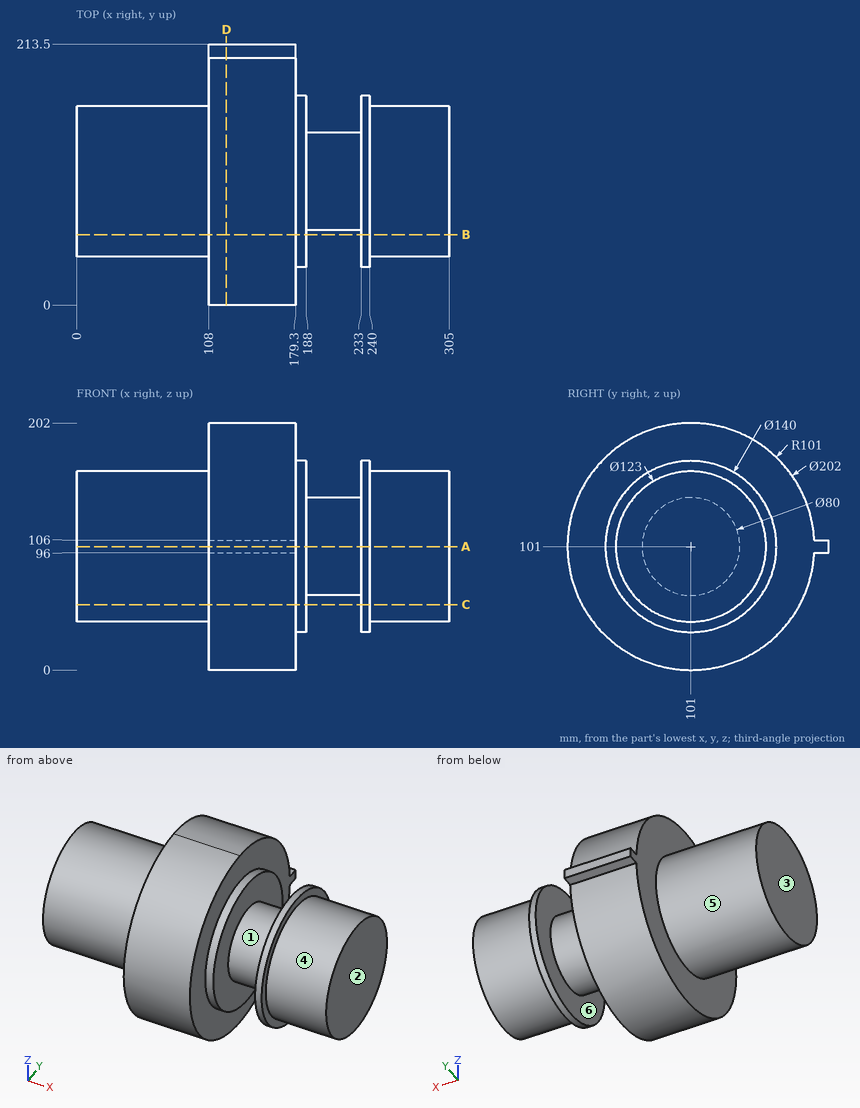
Study the drawing (mm; zero at the part's minimum x, y, z) and answer. A direction names the side the tool comes from. Give positions to 0.01 mm unless a question says otherwise; leave off trailing zeros. Write each loop counter-clockwise with the first axis right and the second up, starting at its lowest first coordinate (ties: lowest second). Pieces come first, ordered by that corner, then holes. Notation, with made-up numbers: (41.25, 76) - (47.25, 76) arc R34 ccw to (47.25, 111) - close; hole circle Ø4 at (33, 23). An arc over 180 degrees is marked (long way). Write item = value, one per line. Start each with the question number.
Item 1: Each of these flat-tipped pins is pushed along its axis until it touches: P1, Ø2, axis at x = 173, y = 171, coming from the -Z side; P2, Ø1, axis at x = 199.5, z = 109, coming from the +Y side; P3, Ø10, axis at x = 112.5, y = 141.5, coming from the +Z side. Where does it stop, or does it pass through?
Item 2: A tool of negligible diameter and unlimited length cuts with its end or side. For the marked faces 4, 5 and 6, from which of +Z, -Z, +X, -X, +Y, -Y can it reach the whole face along a straight path? Write none if from no direction.
Item 3: Find section C-C (z = 53.5). Give the vertices of the cut face in (x, y).
Item 4: Find section A-A (z = 101). Give the vertices of the cut face in (x, y), then the cut area to 3 significant figures.
Item 5: Find section B-B (y = 57.5). Give the vertices of the cut face in (x, z).
Item 6: The mould has two halves that part along X. Classify the marked faces 1, 2 and 3: +X half, -X half, draft (parallel to the pull), parting line (faces both ways), or undercut.
Item 7: Find the intervals of material crossed by probe 1 along X at (y, z) = (42.5, 84); probe 2 along X at (y, z) = (167, 115); probe 3 along X at (y, z) = (17.5, 119), in increasing order. Write a range as [from, to].
Item 8: Find section D-D (x = 122.5). Give the vertices of the cut face in (y, z).
Response:
q1.P1 = 27.24
q1.P2 = 140.29
q1.P3 = 195.56
q2.face_4 = +X
q2.face_5 = -X
q2.face_6 = none
q3.outline = (0, 61.94) - (108, 61.94) - (108, 11.87) - (179.3, 11.87) - (179.3, 49.58) - (188, 49.58) - (188, 152.42) - (179.3, 152.42) - (179.3, 190.13) - (108, 190.13) - (108, 140.06) - (0, 140.06) - close; (233, 49.58) - (240, 49.58) - (240, 61.94) - (305, 61.94) - (305, 140.06) - (240, 140.06) - (240, 152.42) - (233, 152.42) - close
q4.outline = (0, 39.5) - (108, 39.5) - (108, 0) - (179.3, 0) - (179.3, 31) - (188, 31) - (188, 61) - (233, 61) - (233, 31) - (240, 31) - (240, 39.5) - (305, 39.5) - (305, 162.5) - (240, 162.5) - (240, 171) - (233, 171) - (233, 141) - (188, 141) - (188, 171) - (179.3, 171) - (179.3, 213.5) - (108, 213.5) - (108, 162.5) - (0, 162.5) - close
q4.area = 42,300 mm²
q5.outline = (0, 57.53) - (108, 57.53) - (108, 9.85) - (179.3, 9.85) - (179.3, 46.16) - (188, 46.16) - (188, 155.84) - (179.3, 155.84) - (179.3, 192.15) - (108, 192.15) - (108, 144.47) - (0, 144.47) - close; (233, 46.16) - (240, 46.16) - (240, 57.53) - (305, 57.53) - (305, 144.47) - (240, 144.47) - (240, 155.84) - (233, 155.84) - close
q6.face_1 = undercut
q6.face_2 = +X half
q6.face_3 = -X half
q7.probe_1 = [0, 188], [233, 305]
q7.probe_2 = [108, 188], [233, 240]
q7.probe_3 = [108, 179.3]
q8.outline = (201.88, 96) - (213.5, 96) - (213.5, 106) - (201.88, 106) arc R101 ccw (long way) to start
